Part print with two shaded views. Sizes in mm from the minimum x, y, z corner. Round coordinates to 2 decimals unless told otherwise and drop trailing zeros. Loops run counter-clockwise (first coordinate to the right, second up) from the corner with the lowest first, then second, coordinate; pieces in that order, holes last.
(1) Cut at C-C on x = 40.5. List the corners of the cut face in (y, z), then the cut area to 3 significant figures.
(2) Probe probe 1 along Y at (x, z) = (163, 8). List the from-to ranges inside material, lowest first.
(3) Flat gauge pin, fed straight in: pin 1 (5 mm diameter, centred on x = 28, z = 9, fed in from -Y). Where does the tip first touch, or does it go through?
(4) Cut at A-A on z = 6. List the corners of the cut face in (x, y), then the cut area to 3 significant figures.
(5) Cut at B-B on x = 174. List the corners of the cut face in (y, z), then the cut area to 3 significant figures.
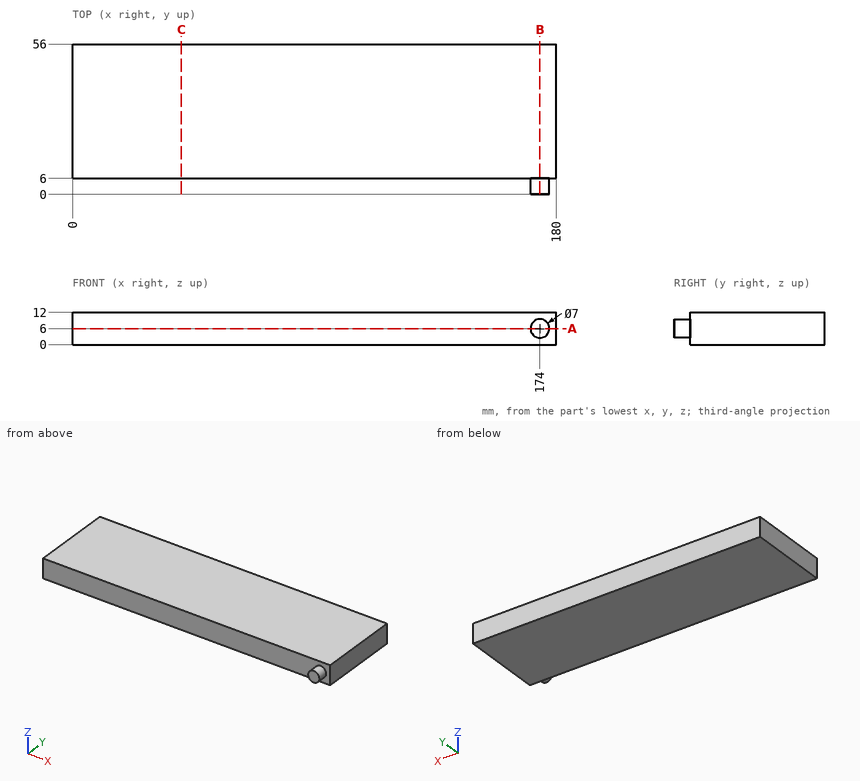
Final values:
1. outline: (6, 0) - (56, 0) - (56, 12) - (6, 12) - close
1. area: 600 mm2
2. probe 1: y = 6 to 56
3. pin 1: stops at y = 6
4. outline: (0, 6) - (170.5, 6) - (170.5, 0) - (177.5, 0) - (177.5, 6) - (180, 6) - (180, 56) - (0, 56) - close
4. area: 9,040 mm2
5. outline: (0, 2.5) - (6, 2.5) - (6, 0) - (56, 0) - (56, 12) - (6, 12) - (6, 9.5) - (0, 9.5) - close
5. area: 642 mm2
